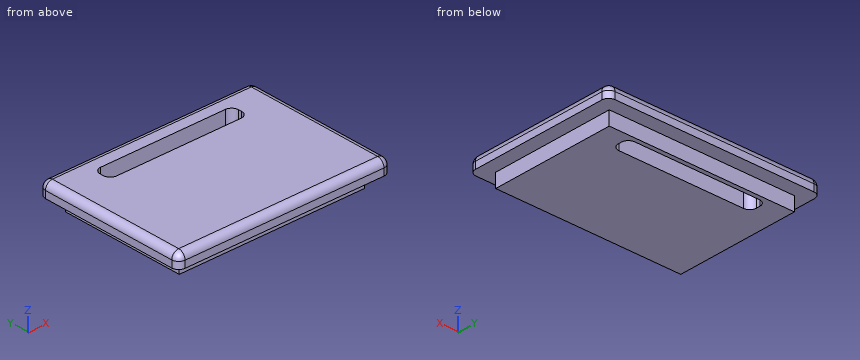
from build123d import *

# Parameters (mm, degrees)
ESQUISSE1_W             = 61.5
ESQUISSE1_H             = 43.75
BOSS_EXTRU_1_DEPTH      = 4
ESQUISSE2_W             = 53.5
ESQUISSE2_H             = 35.75
BOSS_EXTRU_2_DEPTH      = 4
CONG_1_R                = 2
ENL_V_MAT_EXTRU_1_REACH = 10
ESQUISSE3_W             = 40
ESQUISSE3_H             = 5
CONG_2_R                = 2


with BuildPart() as part:
    # Esquisse1 → Boss.-Extru.1 (new body)
    with BuildSketch(Plane.XY):
        with Locations((9.227308767, 0.94004118)):
            Rectangle(ESQUISSE1_W, ESQUISSE1_H)
    extrude(amount=BOSS_EXTRU_1_DEPTH)

    # Esquisse2 → Boss.-Extru.2 (add)
    with BuildSketch(Plane(origin=(0, 0, 0), x_dir=(-1, 0, 0), z_dir=(0, 0, -1))):
        with Locations((-9.227308767, 0.94004118)):
            Rectangle(ESQUISSE2_W, ESQUISSE2_H)
    extrude(amount=BOSS_EXTRU_2_DEPTH)

    # Congé1
    cong_1_edges = [part.edges().sort_by_distance(p)[0] for p in [
        (39.977308767, 0.94004118, 4),
        (9.227308767, 22.81504118, 4),
        (-21.522691233, 0.94004118, 4),
        (-21.522691233, 22.81504118, 2),
        (39.977308767, 22.81504118, 2),
        (39.977308767, -20.93495882, 2),
        (-21.522691233, -20.93495882, 2),
        (9.227308767, -20.93495882, 4),
    ]]
    fillet(cong_1_edges, radius=CONG_1_R)

    # Esquisse3 → Enlèv. mat.-Extru.1 (cut, up to next)
    with BuildSketch(Plane.XY.offset(4), mode=Mode.PRIVATE) as enl_v_mat_extru_1_sk1:
        with Locations((9.477308767, 15.072235538)):
            Rectangle(ESQUISSE3_W, ESQUISSE3_H)
    enl_v_mat_extru_1_tool1 = extrude(enl_v_mat_extru_1_sk1.sketch, amount=-ENL_V_MAT_EXTRU_1_REACH, mode=Mode.PRIVATE) & part.part
    add(enl_v_mat_extru_1_tool1.solids().sort_by_distance((9.477309, 15.072236, 4))[0], mode=Mode.SUBTRACT)

    # Congé2
    cong_2_edges = [part.edges().sort_by_distance(p)[0] for p in [
        (-10.522691233, 12.572235538, 0),
        (-10.522691233, 17.572235538, 0),
        (29.477308767, 17.572235538, 0),
        (29.477308767, 12.572235538, 0),
    ]]
    fillet(cong_2_edges, radius=CONG_2_R)


solid = part.part
For this review, take the finished solid that the model builds, in its own axes (mm). Round coordinates to 2 decimals unless told otherwise and drop trailing zeros. Loops run counter-clockwise (first coordinate to the right, second up) from the corner with the lowest first, then second, coordinate; pieces in that order, holes last. Notation, with made-up numbers: (12.25, 55.25) - (30.25, 55.25) arc R18 ccw to (30.25, 68.25) - close; hole circle Ø9 at (-33.5, 87). An arc over 180 degrees is marked (long way). Put each result on its own line as item: value. Start each with the question number.
1. For probe 1 along Y at (x, z) = (-6, -0.5); probe 2 along Y at (x, z) = (24.5, 1.75); probe 3 along Y at (x, z) = (-17, 2.25), list the stretches that pass through material, from the lowest coordinate up. Write a range as [from, to].
2. Consider section C-C on y = 16.5. State the section outline as (x, z) points, plus the area to 3 significant figures.
3. Insertion check: P1, Ø4.5, axis at y = 1.5, z = -2.5, coming from the +X side; P2, Ø1.5, axis at x = 16, z = 3, coming from the -Y side; P3, Ø4.5, axis at x = 9, z = -2.5, coming from the +Y side. Each pin has a flat end and moves straight along its axis. Give the tip position at first contact, or say it passes through.
4. Consider section D-D on x = 32.5. State the section outline as (y, z) points, plus the area to 3 significant figures.
5. Consider section B-B on x = 19. State the section outline as (y, z) points, plus the area to 3 significant figures.
6. Consider section A-A on z = -0.75. State the section outline as (x, y) points.
Result sheet:
1. probe 1: [-16.93, 12.57], [17.57, 18.82]
1. probe 2: [-20.93, 12.57], [17.57, 22.82]
1. probe 3: [-20.92, 22.8]
2. outline: (-21.52, 0) - (-17.52, 0) - (-17.52, -4) - (-10.29, -4) - (-10.29, 4) - (-19.52, 4) arc R2 ccw to (-21.52, 2) - close; (29.25, -4) - (35.98, -4) - (35.98, 0) - (39.98, 0) - (39.98, 2) arc R2 ccw to (37.98, 4) - (29.25, 4) - close
2. area: 142 mm^2
3. P1: x = 35.98
3. P2: y = -20.92
3. P3: y = 18.82
4. outline: (-20.93, 0) - (-16.93, 0) - (-16.93, -4) - (18.82, -4) - (18.82, 0) - (22.82, 0) - (22.82, 2) arc R2 ccw to (20.82, 4) - (-18.93, 4) arc R2 ccw to (-20.93, 2) - close
4. area: 316 mm^2
5. outline: (-20.93, 0) - (-16.93, 0) - (-16.93, -4) - (12.57, -4) - (12.57, 4) - (-18.93, 4) arc R2 ccw to (-20.93, 2) - close; (17.57, -4) - (18.82, -4) - (18.82, 0) - (22.82, 0) - (22.82, 2) arc R2 ccw to (20.82, 4) - (17.57, 4) - close
5. area: 276 mm^2
6. outline: (-17.52, -16.93) - (35.98, -16.93) - (35.98, 18.82) - (-17.52, 18.82) - close; hole (-10.52, 14.57) arc R2 ccw to (-8.52, 12.57) - (27.48, 12.57) arc R2 ccw to (29.48, 14.57) - (29.48, 15.57) arc R2 ccw to (27.48, 17.57) - (-8.52, 17.57) arc R2 ccw to (-10.52, 15.57) - close
